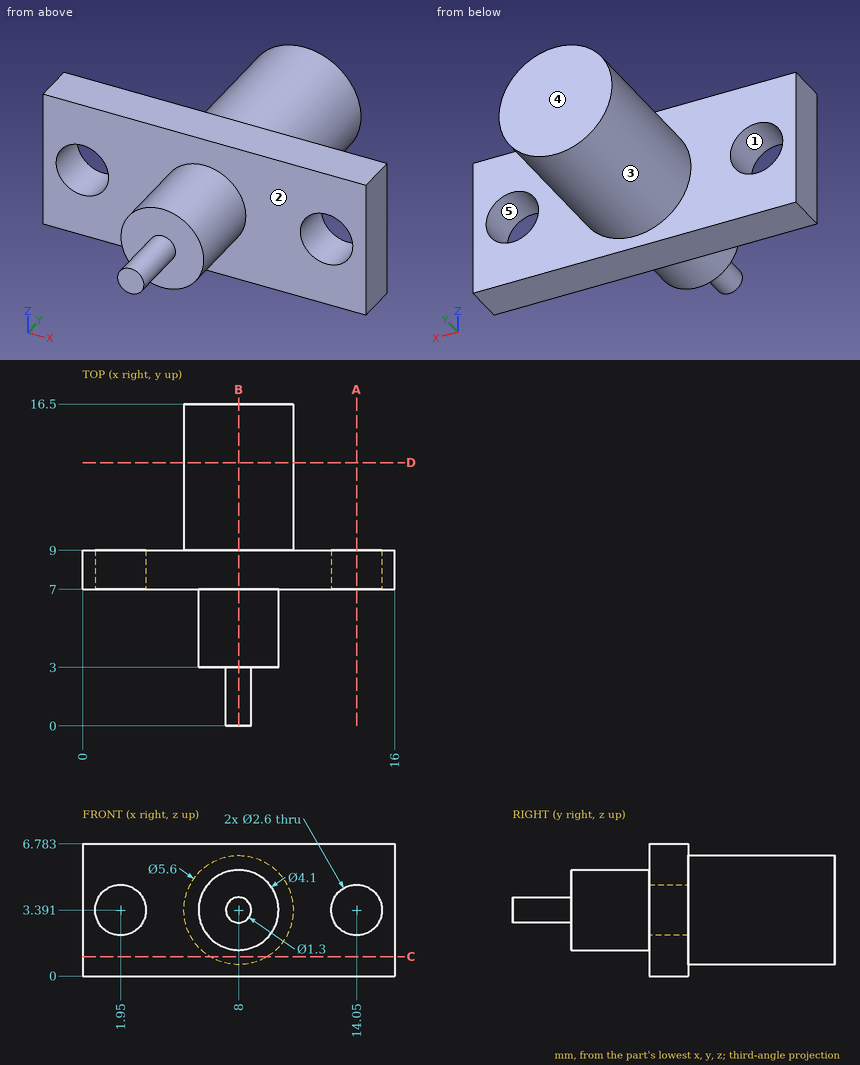
Verification items for this drawing (mm, ordinates from the low corner). A direction names the side the tool comes from. Round coordinates to 2 decimals unless told otherwise and drop trailing zeros. Loops run counter-clockwise (first coordinate to the right, second up) from the corner with the lowest first, then second, coordinate; pieces in that order, holes last. Notation, with made-up numbers: (-7.75, -35.75) - (-3.75, -35.75) arc R20 cw to (-3.75, -2.75) - close; hole circle Ø8 at (-10.75, 15.5). An arc over 180 degrees is marked (long way). Answer as CSV lines item,"result". Start each with the question number.
Item 1: Set-up check for the marked faces 1 and 2: record each of +Z, -Z, +X, -X, +Y, -Y from which the full face is reachable in a straight line by a thin tool's end or side.
Item 2: Section check A-A (x = 14.05). Record the boundary of the cut face in (y, z).
Item 3: Section check D-D (y = 13.5). Record the boundary of the cut face in (x, z), and give its area (3 significant figures).
Item 4: Scan lines: line 1 (X direction, y = 8, z = 4.25) (1 decimal); line 2 (Y direction, x = 13.5, z = 0.5); line 3 (X direction, y = 6, z = 3.25) (1 decimal). Record each from-to range of solid material in increasing order. Write a range as [from, to].
Item 5: Section check C-C (z = 1). Record the boundary of the cut face in (x, y).
Item 6: Depth check by flat-ended pin: P1, Ø3, axis at x = 10, y = 7, coming from the -Z side; P2, Ø1, axis at x = 5, z = 2.5, coming from the -Y side; P3, Ø3.5, axis at x = 1.95, z = 3.39, coming from the +Y side. Enter the tip coordinate at first touch or a pass-through.
Item 7: Section check B-B (x = 8). Record the boundary of the cut face in (y, z).
Item 8: Release check for a two-part mould opening along X. For the marked faces 3, 4 and 5 record: +X half, -X half, draft (parallel to the pull), parting line (faces both ways), or undercut.
Report:
1,face 1,"+Y, -Y"
1,face 2,"-Y"
2,outline,"(7, 0) - (9, 0) - (9, 2.09) - (7, 2.09) - close; (7, 4.69) - (9, 4.69) - (9, 6.78) - (7, 6.78) - close"
3,outline,"circle Ø5.6 at (8, 3.39)"
3,area,"24.6 mm2"
4,line 1,"x = [0, 1], [2.9, 13.1], [15, 16]"
4,line 2,"y = [7, 9]"
4,line 3,"x = [6, 10]"
5,outline,"(0, 7) - (16, 7) - (16, 9) - (9.46, 9) - (9.46, 16.5) - (6.54, 16.5) - (6.54, 9) - (0, 9) - close"
6,P1,"stops at z = 0"
6,P2,"stops at y = 7"
6,P3,"stops at y = 9"
7,outline,"(0, 2.74) - (3, 2.74) - (3, 1.34) - (7, 1.34) - (7, 0) - (9, 0) - (9, 0.59) - (16.5, 0.59) - (16.5, 6.19) - (9, 6.19) - (9, 6.78) - (7, 6.78) - (7, 5.44) - (3, 5.44) - (3, 4.04) - (0, 4.04) - close"
8,face 3,"parting line"
8,face 4,"draft"
8,face 5,"undercut"
